Input: part model. Units: mm. Frame: model coordinates. A direction names the side the tool comes from. Coordinates: 2 decimals unless noted, no trailing zeros. Loops run counter-clockwise (first coordinate to the right, second up) from the corner with the lowest first, then second, coordinate; pieces in that order, holes last.
(1) Contact query for flat-ended pins moving along their axis: P1, Ø0.6, axis at x = 29.5, y = 0.5, coming from the +Z side; P2, Ø0.6, axis at x = 32, y = 1, coming from the -Z side; P3, Ø1.1, axis at y = 1, z = -27.5, coming from the +X side. Output: stop coordinate, or through.
(2) Section B-B, the plane x = -4. Return loops of the section in (y, z).
(3) Line query: L1, parallel to X at y = 0.85, z = 8.5; L2, parallel to Z at x = 3, y = 1.95; L3, parallel to Z at x = 45.5, y = 1. Output: solid intervals per line, ascending.
(4) Section C-C, the plane z = 3.5. Return loops of the section in (x, y).
(5) Section A-A, the plane x = -45. Return loops of the section in (y, z), then the cut area to 3 significant figures.
(6) Set-up query: faces 5 (the face through (-39.43, 0.99, 25.6)), 6 (the face through (-18.859, 0.986, -18.797)), 7 (the face through (40.6, 0.99, -19.43)), 8 (the face through (-49.43, 0.99, 20.6)), 9 (the face through (20.57, 0.99, -25.6)). Return all of +Z, -Z, +X, -X, +Y, -Y with unobstructed straight access to the full face (end or side cutting, diameter ignored); none if empty.
(7) Section D-D, the plane y = 1.35. Give the number of separate pieces and of enclosed holes in the cut face, then the cut area to 3 significant figures.
(8) Mould query, pull axis Z, two halves, no side actions, for faces 1 (the face through (-45, 1, 20)), 2 (the face through (44, 1, 30)), 3 (the face through (46.464, 1.014, -24.675)), 4 (the face through (-50, 1, 24)). Classes: released by +Z, released by -Z, zero draft, split by the parting line, or undercut.
```python
from build123d import *

# Parameters (mm, degrees)
SKETCH_1_W          = 100
SKETCH_1_H          = 60
EXTRUDE_1_DEPTH     = 2
SKETCH_4_W          = 40
SKETCH_4_H          = 40
CUT_EXTRUDE_3_DEPTH = 59.343808583
SKETCH_6_R          = 1.5
CUT_EXTRUDE_5_DEPTH = 59.343808583
SKETCH_7_W          = 20
SKETCH_7_H          = 5
CUT_EXTRUDE_6_DEPTH = 59.343808583
FILLET_1_R          = 4
FILLET_2_R          = 2
SKETCH_8_R          = 1.5
CUT_EXTRUDE_7_DEPTH = 59.343808583
SKETCH_9_W          = 10
SKETCH_9_H          = 40
CUT_EXTRUDE_9_DEPTH = 59.343808583
FILLET_3_R          = 2


with BuildPart() as part:
    # 草图1 → 凸台-拉伸1 (new body)
    with BuildSketch(Plane(origin=(0, 0, 0), x_dir=(1, 0, 0), z_dir=(0, 1, 0))):
        Rectangle(SKETCH_1_W, SKETCH_1_H)
    extrude(amount=EXTRUDE_1_DEPTH)

    # 草图4 → 切除-拉伸3 (cut, through all)
    with BuildSketch(Plane(origin=(0, 2, 0), x_dir=(1, 0, 0), z_dir=(0, 1, 0))):
        Rectangle(SKETCH_4_W, SKETCH_4_H)
    extrude(amount=-CUT_EXTRUDE_3_DEPTH, mode=Mode.SUBTRACT)

    # 草图6 → 切除-拉伸5 (cut, through all)
    with BuildSketch(Plane(origin=(0, 2, 0), x_dir=(1, 0, 0), z_dir=(0, 1, 0))):
        with Locations(Location((-45, 25, 0), (0, 0, 270))):
            Circle(SKETCH_6_R)
        with Locations(Location((-45, -25, 0), (0, 0, 90))):
            Circle(SKETCH_6_R)
        with Locations(Location((45, -25, 0), (0, 0, 270))):
            Circle(SKETCH_6_R)
        with Locations(Location((45, 25, 0), (0, 0, 90))):
            Circle(SKETCH_6_R)
    extrude(amount=-CUT_EXTRUDE_5_DEPTH, mode=Mode.SUBTRACT)

    # 草图7 → 切除-拉伸6 (cut, through all)
    with BuildSketch(Plane(origin=(0, 2, 0), x_dir=(1, 0, 0), z_dir=(0, 1, 0))):
        with Locations((-30, 27.5)):
            Rectangle(SKETCH_7_W, SKETCH_7_H)
        with Locations((-30, -27.5)):
            Rectangle(SKETCH_7_W, SKETCH_7_H)
        with Locations((30, -27.5)):
            Rectangle(SKETCH_7_W, SKETCH_7_H)
        with Locations((30, 27.5)):
            Rectangle(SKETCH_7_W, SKETCH_7_H)
    extrude(amount=-CUT_EXTRUDE_6_DEPTH, mode=Mode.SUBTRACT)

    # 圆角1
    fillet_1_edges = [part.edges().sort_by_distance(p)[0] for p in [
        (20, 1, -20),
        (20, 1, 20),
        (-20, 1, 20),
        (-20, 1, -20),
        (50, 1, 30),
        (-50, 1, 30),
        (-50, 1, -30),
        (50, 1, -30),
    ]]
    fillet(fillet_1_edges, radius=FILLET_1_R)

    # 圆角2
    fillet_2_edges = [part.edges().sort_by_distance(p)[0] for p in [
        (40, 1, -30),
        (40, 1, -25),
        (20, 1, -25),
        (20, 1, -30),
        (40, 1, 30),
        (20, 1, 30),
        (20, 1, 25),
        (40, 1, 25),
        (-40, 1, 30),
        (-40, 1, 25),
        (-20, 1, 25),
        (-20, 1, 30),
        (-40, 1, -25),
        (-40, 1, -30),
        (-20, 1, -30),
        (-20, 1, -25),
    ]]
    fillet(fillet_2_edges, radius=FILLET_2_R)

    # 草图8 → 切除-拉伸7 (cut, through all)
    with BuildSketch(Plane(origin=(0, 2, 0), x_dir=(1, 0, 0), z_dir=(0, 1, 0))):
        with Locations(Location((-15, 25, 0), (0, 0, 270))):
            Circle(SKETCH_8_R)
        with Locations(Location((-15, -25, 0), (0, 0, 90))):
            Circle(SKETCH_8_R)
        with Locations(Location((15, -25, 0), (0, 0, 270))):
            Circle(SKETCH_8_R)
        with Locations(Location((15, 25, 0), (0, 0, 90))):
            Circle(SKETCH_8_R)
    extrude(amount=-CUT_EXTRUDE_7_DEPTH, mode=Mode.SUBTRACT)

    # 草图9 → 切除-拉伸9 (cut, through all)
    with BuildSketch(Plane(origin=(0, 2, 0), x_dir=(1, 0, 0), z_dir=(0, 1, 0))):
        with Locations((-45, 0)):
            Rectangle(SKETCH_9_W, SKETCH_9_H)
        with Locations((45, 0)):
            Rectangle(SKETCH_9_W, SKETCH_9_H)
    extrude(amount=-CUT_EXTRUDE_9_DEPTH, mode=Mode.SUBTRACT)

    # 圆角3
    fillet_3_edges = [part.edges().sort_by_distance(p)[0] for p in [
        (-50, 1, 20),
        (-50, 1, -20),
        (-40, 1, -20),
        (-40, 1, 20),
        (50, 1, -20),
        (50, 1, 20),
        (40, 1, 20),
        (40, 1, -20),
    ]]
    fillet(fillet_3_edges, radius=FILLET_3_R)


solid = part.part
```
Report:
1. P1: stops at z = 25
1. P2: stops at z = -25
1. P3: stops at x = 49.89
2. outline: (0, -30) - (2, -30) - (2, -20) - (0, -20) - close; (0, 20) - (2, 20) - (2, 30) - (0, 30) - close
3. L1: x = -40 to -20, 20 to 40
3. L2: z = -30 to -20, 20 to 30
3. L3: z = -30 to -26.41, -23.59 to -20, 20 to 23.59, 26.41 to 30
4. outline: (-40, 0) - (-20, 0) - (-20, 2) - (-40, 2) - close; (20, 0) - (40, 0) - (40, 2) - (20, 2) - close
5. outline: (0, -30) - (2, -30) - (2, -26.5) - (0, -26.5) - close; (0, -23.5) - (2, -23.5) - (2, -20) - (0, -20) - close; (0, 20) - (2, 20) - (2, 23.5) - (0, 23.5) - close; (0, 26.5) - (2, 26.5) - (2, 30) - (0, 30) - close
5. area: 28.0 mm2
6. face 5: +Z, +Y, -Y
6. face 6: +Y, -Y
6. face 7: +X, +Y, -Y
6. face 8: -X, +Y, -Y
6. face 9: -Z, +Y, -Y
7. separate pieces: 1
7. enclosed holes: 9
7. area: 3,140 mm2
8. face 1: undercut
8. face 2: released by +Z
8. face 3: undercut
8. face 4: zero draft
